from build123d import *

# Parameters (mm, degrees)
F0_R     = 25
F1_DEPTH = 3
F3_DEPTH = 3


with BuildPart() as f1:
    # F0 (on Top) → F1 (new body)
    with BuildSketch(Plane.XY):
        Circle(F0_R)
        with BuildLine():
            add(Edge.make_bspline(
                [(0.9868079036, -7.5640504993), (6.5597245703, -7.5640504993), (6.5597245703, -11.896732791)],
                knots=[0, 0, 0, 1, 1, 1], degree=2))
            add(Edge.make_bspline(
                [(6.5597245703, -11.896732791), (6.5597245703, -14.1558473743), (5.0183834244, -15.3716676868)],
                knots=[0, 0, 0, 1, 1, 1], degree=2))
            add(Edge.make_bspline(
                [(5.0183834244, -15.3716676868), (3.4770422786, -16.5874879993), (0.6092037369, -16.5874879993)],
                knots=[0, 0, 0, 1, 1, 1], degree=2))
            Line((0.6092037369, -16.5874879993), (-1.1420983464, -16.5874879993))
            Line((-1.1420983464, -16.5874879993), (-1.1420983464, -22.4370973743))
            Line((-1.1420983464, -22.4370973743), (-2.8706139714, -22.4370973743))
            Line((-2.8706139714, -22.4370973743), (-2.8706139714, -7.5640504993))
            Line((-2.8706139714, -7.5640504993), (0.9868079036, -7.5640504993))
        make_face(mode=Mode.SUBTRACT)
    extrude(amount=F1_DEPTH)



with BuildPart() as f1b:
    # F0 (on Top) → F1, piece 2 (new body)
    with BuildSketch(Plane.XY):
        with BuildLine():
            Line((-1.1420983464, -9.0614463327), (-1.1420983464, -15.1031129993))
            Line((-1.1420983464, -15.1031129993), (0.4171464453, -15.1031129993))
            add(Edge.make_bspline(
                [(0.4171464453, -15.1031129993), (2.7153235286, -15.1031129993), (3.7423417578, -14.3609254993)],
                knots=[0, 0, 0, 1, 1, 1], degree=2))
            add(Edge.make_bspline(
                [(3.7423417578, -14.3609254993), (4.7693599869, -13.6187379993), (4.7693599869, -11.9781129993)],
                knots=[0, 0, 0, 1, 1, 1], degree=2))
            add(Edge.make_bspline(
                [(4.7693599869, -11.9781129993), (4.7693599869, -10.5035036243), (3.8025631119, -9.7824749785)],
                knots=[0, 0, 0, 1, 1, 1], degree=2))
            add(Edge.make_bspline(
                [(3.8025631119, -9.7824749785), (2.8357662369, -9.0614463327), (0.7914954036, -9.0614463327)],
                knots=[0, 0, 0, 1, 1, 1], degree=2))
            Line((0.7914954036, -9.0614463327), (-1.1420983464, -9.0614463327))
        make_face()
    extrude(amount=F1_DEPTH)


with BuildPart() as f1_1:
    add(f1.part)

    add(f1b.part)  # F3 merges F1b
    # F2 (on Top) → F3 (join)
    with BuildSketch(Plane.XY):
        Polygon((0, -10.621725142), (-9.7534448872, -10.621725142), (-9.6736760242, -13.621725142), (0, -13.621725142), align=None)
    extrude(amount=F3_DEPTH)


solid = f1_1.part
Geometry check sheet. Reference: the model listing, model coordinates, mm. A direction names the side the tool comes from. Round coordinates to 2 decimals unless told otherwise and drop trailing zeros. Write each loop counter-clockwise with the first axis right and the second up, starting at its lowest first coordinate (ties: lowest second). Pieces come first, ordered by that corner, then holes.
Item 1: Section check C-C (y = 20). Record the boundary of the cut face in (x, z).
Determined:
outline: (-15, 0) - (15, 0) - (15, 3) - (-15, 3) - close
Item 2: Section check A-A (x = -2). Record the boundary of the cut face in (y, z), plus the area to 3 significant figures.
Determined:
outline: (-24.92, 0) - (-22.44, 0) - (-22.44, 3) - (-24.92, 3) - close; (-13.62, 0) - (-10.62, 0) - (-10.62, 3) - (-13.62, 3) - close; (-7.56, 0) - (24.92, 0) - (24.92, 3) - (-7.56, 3) - close
area: 114 mm2
Item 3: Section check B-B (y = -20.5). Record the boundary of the cut face in (x, z).
Determined:
outline: (-14.31, 0) - (-2.87, 0) - (-2.87, 3) - (-14.31, 3) - close; (-1.14, 0) - (14.31, 0) - (14.31, 3) - (-1.14, 3) - close
Item 4: Access from +Z, -Z, +X, -X, +Y, -Y to the whole of each face (thin tool, end or side, straight path). Record for faces 1 (the face through (-2.871, -9, 1)), 2 (the face through (0, 0, 3)).
Determined:
face 1: +Z, -Z
face 2: +Z, +X, -X, +Y, -Y
Item 5: Material ranges on line 1 along Y through (x, z) = (0.5, 2.75) (3 decimals); line 2 along X through (y, z) = (-22, 1); line 3 along Y through (x, z) = (6, 0.8), recorded low to high.
Determined:
line 1: y = -24.995 to -16.587, -15.103 to -9.061, -7.564 to 24.995
line 2: x = -11.87 to -2.87, -1.14 to 11.87
line 3: y = -24.27 to -14.24, -9.59 to 24.27
Item 6: Section check D-D (x = -10). Record the boundary of the cut face in (y, z).
Determined:
outline: (-22.91, 0) - (22.91, 0) - (22.91, 3) - (-22.91, 3) - close
Item 7: Mould release check, pull along Y, two halves, no side actions. Record for faces 3 (the face through (23.846, 7.509, 1.479)), 4 (the face through (0, 0, 0)), 5 (the face through (-1.142, -19, 1)), 6 (the face through (-2.871, -18, 1)): +Y half, -Y half, draft (parallel to the pull), parting line (faces both ways), or undercut.
Determined:
face 3: parting line
face 4: draft
face 5: undercut
face 6: undercut
Item 8: Go/stop test with flat-tipped pins: pin 1 Ø1.5 at (y, z) = (-8.5, 1.5) entering from +X; pin 2 Ø1.4 at (x, z) = (-1.5, 1.5) entering from -Y; pin 3 Ø0.9 at (y, z) = (-20, 1.5) entering from +X. Record where each tip stops, or that it passes through.
Determined:
pin 1: stops at x = 23.77
pin 2: stops at y = -24.99
pin 3: stops at x = 15.58
